from build123d import *

# Parameters (mm, degrees)
SKETCH_W        = 20
SKETCH_H        = 14
PAD_DEPTH       = 20
SKETCH001_W     = 10
SKETCH001_H     = 14
POCKET_DEPTH    = 5
SKETCH002_R     = 1.6
POCKET001_DEPTH = 20
SKETCH003_R     = 4
POCKET002_DEPTH = 10


with BuildPart() as part:
    # Sketch → Pad (new body)
    with BuildSketch(Plane.XY):
        with Locations((10, 7)):
            Rectangle(SKETCH_W, SKETCH_H)
    extrude(amount=PAD_DEPTH)

    # Sketch001 (on Face6 of Pad) → Pocket (cut)
    with BuildSketch(Plane.XY.offset(20)):
        with Locations((5, 7)):
            Rectangle(SKETCH001_W, SKETCH001_H)
    extrude(amount=-POCKET_DEPTH, mode=Mode.SUBTRACT)

    # Sketch002 (on Face4 of Pocket) → Pocket001 (cut)
    with BuildSketch(Plane.XY.offset(20)):
        with Locations((15, 7)):
            Circle(SKETCH002_R)
    extrude(amount=-POCKET001_DEPTH, mode=Mode.SUBTRACT)

    # Sketch003 (on Face4 of Pocket001) → Pocket002 (cut)
    with BuildSketch(Plane.XY.offset(20)):
        with Locations((15, 7)):
            Circle(SKETCH003_R)
    extrude(amount=-POCKET002_DEPTH, mode=Mode.SUBTRACT)


solid = part.part
Build history of the part. All positions in model axes, mm. A direction names the side the tool comes from. Give positions to 0.01 mm unless a question says otherwise; leave off trailing zeros. Order: outer loops, then holes, each group sorted by start corner. A loop starts at its lowest first (then second) coordinate and runs counter-clockwise, first axis right, second up. Notation, with made-up numbers: M -2.75,24.25 L 16.25,24.25 A23 ccw 16.25,45.25 Z; hole C 83.5,6 d1. An arc over 180 degrees is marked long. Use one line per item in the form item = value.
1) Drop flat-ended pins along their axis: pin 1 (5.5 mm diameter, centred on y = 3.5, z = 18, fed in from -X); pin 2 (5 mm diameter, centred on x = 7, y = 7.5, fed in from +Z). Give the stop position or say it passes through.
Calculated:
pin_1 = 10
pin_2 = 15
2) Saw through at A-A (y = 7). Give the cut face in (x, z), plus the area to 3 significant figures.
Calculated:
outline = M 0,0 L 13.4,0 L 13.4,10 L 11,10 L 11,20 L 10,20 L 10,15 L 0,15 Z; M 16.6,0 L 20,0 L 20,20 L 19,20 L 19,10 L 16.6,10 Z
area = 238 mm2
3) Two-plate mould, pull along X, no slides. Class faces 4 (the face through (20, 7, 10)), 5 (the face through (0, 7, 7)), 6 (the face through (10.5, 7.1, 20)), 7 (the face through (15, 5, 10)): released by +X, released by -X, zero draft, split by the parting line, or undercut.
Calculated:
face_4 = released by +X
face_5 = released by -X
face_6 = zero draft
face_7 = undercut
4) Probe probe 1 along Y at (x, z) = (15, 4); probe 2 along Y at (x, z) = (15, 15.75); probe 3 along Z at (x, y) = (6.5, 9.75). List the from-to ranges inside material, lowest first.
Calculated:
probe_1 = 0 to 5.4, 8.6 to 14
probe_2 = 0 to 3, 11 to 14
probe_3 = 0 to 15
5) Tool access for faces 1 (the face through (10, 7, 0)), 2 (the face through (11, 7, 15)), 3 (the face through (10, 7, 18)): list every direction of +Z, -Z, +X, -X, +Y, -Y with a clear straight run to the whole face (end or side of a thin tool).
Calculated:
face_1 = -Z, +X, -X, +Y, -Y
face_2 = +Z
face_3 = +Z, -X, +Y, -Y
6) Saw through at B-B (x = 15). Give the cut face in (y, z), plus the area to 3 significant figures.
Calculated:
outline = M 0,0 L 5.4,0 L 5.4,10 L 3,10 L 3,20 L 0,20 Z; M 8.6,0 L 14,0 L 14,20 L 11,20 L 11,10 L 8.6,10 Z
area = 168 mm2
7) Saw through at D-D (y = 12.5). Give the cut face in (x, z), plus the area to 3 significant figures.
Calculated:
outline = M 0,0 L 20,0 L 20,20 L 10,20 L 10,15 L 0,15 Z
area = 350 mm2
8) Saw through at C-C (z = 13). Give the cut face in (x, y).
Calculated:
outline = M 0,0 L 20,0 L 20,14 L 0,14 Z; hole C 15,7 d8
